from build123d import *
from OCP.BRepFilletAPI import BRepFilletAPI_MakeChamfer

# Parameters (mm, degrees)
SKETCH1_R             = 1.7
BOSS_EXTRUDE1_DEPTH   = 2
SKETCH2_W             = 30
SKETCH2_H             = 2
BOSS_EXTRUDE2_DEPTH   = 35
CUT_EXTRUDE1_DEPTH    = 2
SKETCH5_W             = 17
SKETCH5_H             = 15.5
CUT_EXTRUDE2_DEPTH    = 2
SKETCH6_R             = 1.2
CUT_EXTRUDE3_DEPTH    = 2
BOSS_EXTRUDE4_START   = -2
SKETCH7_W             = 30
SKETCH7_H             = 2
BOSS_EXTRUDE4_DEPTH   = 2
SKETCH8_W             = 20
SKETCH8_H             = 3
CUT_EXTRUDE4_DEPTH    = 2
SKETCH9_W             = 17
SKETCH9_H             = 3
CUT_EXTRUDE5_DEPTH    = 2
SKETCH10_W            = 2
SKETCH10_H            = 20
BOSS_EXTRUDE5_DEPTH   = 5
CUT_EXTRUDE6_START    = -30
CUT_EXTRUDE6_DEPTH    = 30
FILLET1_R             = 10
SKETCH12_W            = 20
SKETCH12_H            = 18.563508327
CUT_EXTRUDE7_DEPTH    = 2
FILLET2_R             = 2
BOSS_EXTRUDE6_START   = -2
BOSS_EXTRUDE6_DEPTH   = 2
BOSS_EXTRUDE7_START   = -2
SKETCH14_W            = 21
SKETCH14_H            = 11.5
BOSS_EXTRUDE7_DEPTH   = 2
BOSS_EXTRUDE8_START   = -2
BOSS_EXTRUDE8_DEPTH   = 2
FILLET3_R             = 2
FILLET4_R             = 6
SKETCH16_W            = 20
SKETCH16_H            = 8.5
CUT_EXTRUDE8_DEPTH    = 2
FILLET5_R             = 5
CHAMFER1_SIZE         = 2
CHAMFER1_SIZE2        = 2.748737084
CHAMFER1_SIZE2_2      = 2.596624047
CHAMFER2_SIZE         = 1
CHAMFER2_EDGE_2_SIZE  = 1
CHAMFER2_EDGE_3_SIZE  = 1
CHAMFER2_EDGE_3_SIZE2 = 2.732050808
CHAMFER2_EDGE_4_SIZE  = 1
CHAMFER2_EDGE_4_SIZE2 = 2.732050808
FILLET6_R             = 6


# Some blends are built 0.0001 mm under size
with BuildPart() as part:
    # Sketch1 → Boss-Extrude1 (new body)
    with BuildSketch(Plane(origin=(0, 0, 0), x_dir=(1, 0, 0), z_dir=(0, 1, 0))):
        with BuildLine():
            Line((-21.310608918, 0), (21.310608918, 0))
            ThreePointArc((21.310608918, 0), (26.45, 5.139391082), (31.589391082, 0))
            Line((31.589391082, 0), (31.589391082, -16))
            Line((31.589391082, -16), (10, -16))
            Line((10, -16), (10, -10.526162893))
            Line((10, -10.526162893), (10, -3))
            Line((10, -3), (-10, -3))
            Line((-10, -3), (-10, -10.526162893))
            Line((-10, -10.526162893), (-10, -16))
            Line((-10, -16), (-31.589391082, -16))
            Line((-31.589391082, -16), (-31.589391082, 0))
            ThreePointArc((-31.589391082, 0), (-26.45, 5.139391082), (-21.310608918, 0))
        make_face()
        with Locations(Location((-26.45, 0, 0), (0, 0, 270))):
            Circle(SKETCH1_R, mode=Mode.SUBTRACT)
        with Locations(Location((26.45, 0, 0), (0, 0, 270))):
            Circle(SKETCH1_R, mode=Mode.SUBTRACT)
    extrude(amount=BOSS_EXTRUDE1_DEPTH)

    # Sketch2 → Boss-Extrude2 (add)
    with BuildSketch(Plane(origin=(0, 2, 0), x_dir=(1, 0, 0), z_dir=(0, 1, 0))):
        with Locations((0, -15)):
            Rectangle(SKETCH2_W, SKETCH2_H)
    extrude(amount=BOSS_EXTRUDE2_DEPTH)

    # Sketch4 → Cut-Extrude1 (cut)
    with BuildSketch(Plane.XY.offset(16)):
        with BuildLine():
            Line((-12.5, 33), (-12.5, 24.5))
            Line((-12.5, 24.5), (-10.5, 24.5))
            ThreePointArc((-10.5, 24.5), (-9.085786438, 23.914213562), (-8.5, 22.5))
            Line((-8.5, 22.5), (-8.5, 20.5))
            Line((-8.5, 20.5), (8.5, 20.5))
            Line((8.5, 20.5), (8.5, 22.5))
            ThreePointArc((8.5, 22.5), (9.085786438, 23.914213562), (10.5, 24.5))
            Line((10.5, 24.5), (12.5, 24.5))
            Line((12.5, 24.5), (12.5, 33))
            Line((12.5, 33), (10.5, 33))
            ThreePointArc((10.5, 33), (9.085786438, 33.585786438), (8.5, 35))
            Line((8.5, 35), (8.5, 37))
            Line((8.5, 37), (-8.5, 37))
            Line((-8.5, 37), (-8.5, 35))
            ThreePointArc((-8.5, 35), (-9.085786438, 33.585786438), (-10.5, 33))
            Line((-10.5, 33), (-12.5, 33))
        make_face()
    extrude(amount=-CUT_EXTRUDE1_DEPTH, mode=Mode.SUBTRACT)

    # Sketch5 → Cut-Extrude2 (cut)
    with BuildSketch(Plane.XY.offset(16)):
        with Locations((0, 12.75)):
            Rectangle(SKETCH5_W, SKETCH5_H)
    extrude(amount=-CUT_EXTRUDE2_DEPTH, mode=Mode.SUBTRACT)

    # Sketch6 → Cut-Extrude3 (cut)
    with BuildSketch(Plane.XY.offset(16)):
        with Locations((-10.5, 35)):
            Circle(SKETCH6_R)
        with Locations((10.5, 35)):
            Circle(SKETCH6_R)
        with Locations((-10.5, 22.5)):
            Circle(SKETCH6_R)
        with Locations((10.5, 22.5)):
            Circle(SKETCH6_R)
    extrude(amount=-CUT_EXTRUDE3_DEPTH, mode=Mode.SUBTRACT)

    # Sketch7 → Boss-Extrude4 (add)
    with BuildSketch(Plane.XY.offset(16).offset(BOSS_EXTRUDE4_START)):
        with Locations((0, 38)):
            Rectangle(SKETCH7_W, SKETCH7_H)
    extrude(amount=BOSS_EXTRUDE4_DEPTH)

    # Sketch8 → Cut-Extrude4 (cut)
    with BuildSketch(Plane(origin=(0, 2, 0), x_dir=(1, 0, 0), z_dir=(0, 1, 0))):
        with Locations((0, -1.5)):
            Rectangle(SKETCH8_W, SKETCH8_H)
    extrude(amount=-CUT_EXTRUDE4_DEPTH, mode=Mode.SUBTRACT)

    # Sketch9 → Cut-Extrude5 (cut)
    with BuildSketch(Plane.XY.offset(16)):
        with Locations((0, 3.5)):
            Rectangle(SKETCH9_W, SKETCH9_H)
    extrude(amount=-CUT_EXTRUDE5_DEPTH, mode=Mode.SUBTRACT)

    # Sketch10 → Boss-Extrude5 (add)
    with BuildSketch(Plane(origin=(0, 0, 14), x_dir=(-1, 0, 0), z_dir=(0, 0, -1))):
        with Locations((14, 12)):
            Rectangle(SKETCH10_W, SKETCH10_H)
        with Locations((-14, 12)):
            Rectangle(SKETCH10_W, SKETCH10_H)
    extrude(amount=BOSS_EXTRUDE5_DEPTH)

    # Sketch11 → Cut-Extrude6 (cut)
    with BuildSketch(Plane.ZY.offset(15).offset(CUT_EXTRUDE6_START)):
        Polygon((14, 22), (9, 2), (9, 22), align=None)
    extrude(amount=CUT_EXTRUDE6_DEPTH, mode=Mode.SUBTRACT)

    # Fillet1
    fillet1_edges = [part.edges().sort_by_distance(p)[0] for p in [
        (31.589391082, 1, 16),
        (-31.589391082, 1, 16),
    ]]
    fillet(fillet1_edges, radius=FILLET1_R)

    # Sketch12 → Cut-Extrude7 (cut)
    with BuildSketch(Plane.XY.offset(16)):
        with Locations((0, 11.281754164)):
            Rectangle(SKETCH12_W, SKETCH12_H)
    extrude(amount=-CUT_EXTRUDE7_DEPTH, mode=Mode.SUBTRACT)

    # Fillet2
    # the kernel refuses this fillet: 2 mm, written as the material it takes off along each edge
    with BuildSketch(Plane(origin=(8.5, 20.563508327, 9.158770817), x_dir=(0, 1, 0), z_dir=(0, 0, 1))) as fillet2_piece_1:
        with BuildLine():
            CenterArc((1.936491673, -2), FILLET2_R, 90, 75.522487814)
            Line((0, -1.5), (-0.038729833, -1.49))
            ThreePointArc((-0.038729833, -1.49), (-0.04, -0.75), (-0.04, 0))
            Line((-0.04, 0), (0, 0.04))
            Line((0, 0.04), (1.936491673, 0.04))
            Line((1.936491673, 0.04), (1.936491673, 0))
        make_face()
    extrude(amount=11.682458366, mode=Mode.SUBTRACT)
    with BuildSketch(Plane(origin=(-8.5, 20.563508327, 9.158770817), x_dir=(-1, 0, 0), z_dir=(0, 0, 1))) as fillet2_piece_2:
        with BuildLine():
            CenterArc((2, -1.936491673), FILLET2_R, 104.477512186, 75.522487814)
            Line((0, -1.936491673), (-0.04, -1.936491673))
            Line((-0.04, -1.936491673), (-0.04, 0))
            Line((-0.04, 0), (0, 0.04))
            ThreePointArc((0, 0.04), (0.75, 0.04), (1.49, 0.038729833))
            Line((1.49, 0.038729833), (1.5, 0))
        make_face()
    extrude(amount=11.682458366, mode=Mode.SUBTRACT)

    # Sketch13 → Boss-Extrude6 (add)
    with BuildSketch(Plane.XY.offset(16).offset(BOSS_EXTRUDE6_START)):
        Polygon((-15, 2), (-15, 33), (-21.589391082, 2), align=None)
        Polygon((21.589391082, 2), (15, 2), (15, 33), align=None)
    extrude(amount=BOSS_EXTRUDE6_DEPTH)

    # Sketch14 → Boss-Extrude7 (add)
    with BuildSketch(Plane.XY.offset(16).offset(BOSS_EXTRUDE7_START)):
        with Locations((0, 10.75)):
            Rectangle(SKETCH14_W, SKETCH14_H)
    extrude(amount=BOSS_EXTRUDE7_DEPTH)

    # Sketch15 → Boss-Extrude8 (add)
    with BuildSketch(Plane.XY.offset(16).offset(BOSS_EXTRUDE8_START)):
        with BuildLine():
            Line((-8.5, 22.5), (-8.5, 16.5))
            Line((-8.5, 16.5), (-10, 16.5))
            Line((-10, 16.5), (-10, 20.563508327))
            ThreePointArc((-10, 20.563508327), (-8.91886117, 21.275255129), (-8.5, 22.5))
        make_face()
        with BuildLine():
            Line((8.5, 22.5), (8.5, 16.5))
            Line((8.5, 16.5), (10, 16.5))
            Line((10, 16.5), (10, 20.563508327))
            ThreePointArc((10, 20.563508327), (8.91886117, 21.275255129), (8.5, 22.5))
        make_face()
    extrude(amount=BOSS_EXTRUDE8_DEPTH)

    # Fillet3
    fillet3_edges = [part.edges().sort_by_distance(p)[0] for p in [
        (-8.5, 16.5, 15),
        (8.5, 16.5, 15),
        (12.5, 24.5, 15),
        (-12.5, 24.5, 15),
        (12.5, 33, 15),
        (8.5, 37, 15),
        (-8.5, 37, 15),
        (-12.5, 33, 15),
    ]]
    fillet(fillet3_edges, radius=FILLET3_R - 0.0001)  # a hair under: the kernel refuses the full size

    # Fillet4
    fillet4_edges = [part.edges().sort_by_distance(p)[0] for p in [
        (15, 39, 15),
        (-15, 39, 15),
    ]]
    fillet(fillet4_edges, radius=FILLET4_R - 0.0001)  # a hair under: the kernel refuses the full size

    # Sketch16 → Cut-Extrude8 (cut)
    with BuildSketch(Plane.XY.offset(16)):
        with Locations((0, 9.25)):
            Rectangle(SKETCH16_W, SKETCH16_H)
    extrude(amount=-CUT_EXTRUDE8_DEPTH, mode=Mode.SUBTRACT)

    # Fillet5
    fillet5_edges = [part.edges().sort_by_distance(p)[0] for p in [
        (-10, 13.5, 15),
        (10, 13.5, 15),
    ]]
    fillet(fillet5_edges, radius=FILLET5_R)

    # Chamfer1: one chamfer whose edges measure the first distance from different faces: ONE call of the kernel's chamfer builder (chamfer() names one face for all edges)
    chamfer1_edges_1 = [part.edges().sort_by_distance(p)[0] for p in [
        (-13, 2, 11.5),
        (11.5, 2, 14),
        (13, 2, 11.5),
        (-18.294695541, 2, 14),
        (15, 2, 11.5),
        (18.294695541, 2, 14),
        (-11.5, 2, 14),
        (-15, 2, 11.5),
    ]]
    chamfer1_edges_2 = [part.edges().sort_by_distance(p)[0] for p in [
        (-14, 2, 9),
    ]]
    chamfer1_side_2 = [part.faces().sort_by_distance(p)[0] for p in [
        (-21.362181676, 2, 5.92457091),
    ]]
    chamfer1_edges_3 = [part.edges().sort_by_distance(p)[0] for p in [
        (14, 2, 9),
    ]]
    chamfer1_side_3 = [part.faces().sort_by_distance(p)[0] for p in [
        (21.362181676, 2, 5.92457091),
    ]]
    chamfer1_edges_4 = [part.edges().sort_by_distance(p)[0] for p in [
        (-21.589391082, 2, 15),
    ]]
    chamfer1_side_4 = [part.faces().sort_by_distance(p)[0] for p in [
        (-21.362181676, 2, 5.92457091),
    ]]
    chamfer1_edges_5 = [part.edges().sort_by_distance(p)[0] for p in [
        (21.589391082, 2, 15),
    ]]
    chamfer1_side_5 = [part.faces().sort_by_distance(p)[0] for p in [
        (18.294695541, 17.5, 15),
    ]]
    chamfer1 = BRepFilletAPI_MakeChamfer(part.part.solid().wrapped)
    for e in chamfer1_edges_1:
        chamfer1.Add(CHAMFER1_SIZE, e.wrapped)
    for e in chamfer1_edges_2:
        chamfer1.Add(CHAMFER1_SIZE, CHAMFER1_SIZE2, e.wrapped, chamfer1_side_2[0].wrapped)  # the first distance lies on this face
    for e in chamfer1_edges_3:
        chamfer1.Add(CHAMFER1_SIZE, CHAMFER1_SIZE2, e.wrapped, chamfer1_side_3[0].wrapped)  # the first distance lies on this face
    for e in chamfer1_edges_4:
        chamfer1.Add(CHAMFER1_SIZE, CHAMFER1_SIZE2_2, e.wrapped, chamfer1_side_4[0].wrapped)  # the first distance lies on this face
    for e in chamfer1_edges_5:
        chamfer1.Add(CHAMFER1_SIZE, CHAMFER1_SIZE2_2, e.wrapped, chamfer1_side_5[0].wrapped)  # the first distance lies on this face
    add(Compound.cast(chamfer1.Shape()), mode=Mode.REPLACE)

    # Chamfer2
    chamfer2_edges = [part.edges().sort_by_distance(p)[0] for p in [
        (15, 13, 14),
    ]]
    chamfer(chamfer2_edges, length=CHAMFER2_SIZE)

    # Chamfer2 edge 2
    chamfer2_edge_2_edges = [part.edges().sort_by_distance(p)[0] for p in [
        (-15, 13, 14),
    ]]
    chamfer(chamfer2_edge_2_edges, length=CHAMFER2_EDGE_2_SIZE)

    # Chamfer2 edge 3
    chamfer2_edge_3_edges = [part.edges().sort_by_distance(p)[0] for p in [
        (16, 3, 13),
    ]]
    chamfer2_edge_3_side = [part.faces().sort_by_distance(p)[0] for p in [
        (19.357625286, 2.973019207, 12.973019207),
    ]]
    chamfer(chamfer2_edge_3_edges, length=CHAMFER2_EDGE_3_SIZE, length2=CHAMFER2_EDGE_3_SIZE2, reference=chamfer2_edge_3_side[0])

    # Chamfer2 edge 4
    chamfer2_edge_4_edges = [part.edges().sort_by_distance(p)[0] for p in [
        (-16, 3, 13),
    ]]
    chamfer2_edge_4_side = [part.faces().sort_by_distance(p)[0] for p in [
        (-19.294695541, 3, 13),
    ]]
    chamfer(chamfer2_edge_4_edges, length=CHAMFER2_EDGE_4_SIZE, length2=CHAMFER2_EDGE_4_SIZE2, reference=chamfer2_edge_4_side[0])

    # Fillet6
    fillet6_edges = [part.edges().sort_by_distance(p)[0] for p in [
        (-10, 1, 0),
        (10, 1, 0),
    ]]
    fillet(fillet6_edges, radius=FILLET6_R)


solid = part.part
CAD build for the part. Positions are in the model's coordinates, mm. A direction names the side the tool comes from. Coordinates: 2 decimals unless noted, no trailing zeros. Write each loop counter-clockwise with the first axis right and the second up, starting at its lowest first coordinate (ties: lowest second). Pieces come first, ordered by that corner, then holes. Notation, with made-up numbers: (55, 2) - (90, 2) arc R34 cw to (90, 34) - close; hole circle Ø2 at (82, 2.5). An arc over 180 degrees is marked (long way). Use a Markdown table: item, result. Add a question column.
Item 1: Drill centre lines: L1, parallel to Y at x = -10.5, z = 15.5; L2, parallel to Z at x = -18, y = 13.5; L3, parallel to Y at x = -11, z = 7. Where is each one in solid material? Low to high. Write a range as from..to.
Item 2: Flat gauge pins, fed straight in: pin 1 (10 mm diameter, centred on x = -3, y = 6.5, fed in from -Z); pin 2 (3 mm diameter, centred on x = -10.5, y = 35, fed in from +Z); pin 3 (1.6 mm diameter, centred on y = 29.5, z = 14.5, fed in from +X); pin 4 (2 mm diameter, centred on x = 19, y = 1, fed in from -Z). Where does each tip first touch, or does it go through?
Item 3: Band-saw the part on B-B, the plane y = 6. Give the cut face in (x, z).
Item 4: 3-axis set-ups, long thin cutter, end or side, ignore diameter. For faces 5 (the face through (-13, 9, 13)), 6 (the face through (0, 13.5, 15)), 7 (the face through (-7.93, 17.1, 15.01)), 8 (the face through (13.196, 37.289, 15.014)): which of +Z, -Z, +X, -X, +Y, -Y reach the whole face in a straight line?
Item 5: Mould opens along X. For faces 1 (the face through (-11.9, 25.07, 14.99)), 2 (the face through (-13.289, 37.196, 15.014)), 3 (the face through (-11.711, 0.986, 1.804)), 4 (the face through (22.701, 2.964, 14.416)) say: pulls with the +X half, pulls with the -X half, needs draft (parallel to the pull), parting line crosses it, or undercut.
Item 6: Band-saw the part on D-D, the plane x = -26.45. Give the cut face in (y, z), and give its area (3 significant figures).
Item 7: Band-saw the part on A-A, the plane x = -1. Give the cut face in (y, z), and give its area (3 significant figures).
Item 8: Band-saw the part on C-C, the plane y = 10.5. Give the cut face in (x, z) (3 decimals).
Numbers:
| question | item | result |
|---|---|---|
| 1 | L1 | 0..21.3, 23.7..24.5, 33..33.8, 36.2..38.81 |
| 1 | L2 | 14..16 |
| 1 | L3 | 0..2 |
| 2 | pin 1 | through |
| 2 | pin 2 | z = 16 |
| 2 | pin 3 | x = 15.91 |
| 2 | pin 4 | z = 0 |
| 3 | outline | (-20.74, 14) - (-16, 14) - (-15, 13) - (-15, 10) - (-13, 10) - (-13, 14) - (-10, 14) - (-10, 16) - (-20.74, 16) - close; (10, 14) - (13, 14) - (13, 10) - (15, 10) - (15, 13) - (16, 14) - (20.74, 14) - (20.74, 16) - (10, 16) - close |
| 4 | face 5 | -Z, +Y |
| 4 | face 6 | +Z, -Z, -Y |
| 4 | face 7 | +Z, -Z |
| 4 | face 8 | +Z, -Z, +X, +Y |
| 5 | face 1 | undercut |
| 5 | face 2 | pulls with the -X half |
| 5 | face 3 | undercut |
| 5 | face 4 | pulls with the +X half |
| 6 | outline | (0, -5.14) - (2, -5.14) - (2, -1.7) - (0, -1.7) - close; (0, 1.7) - (2, 1.7) - (2, 14.74) - (0, 14.74) - close |
| 6 | area | 33.0 mm2 |
| 7 | outline | (13.5, 14) - (16.5, 14) - (16.5, 16) - (13.5, 16) - close; (37, 14) - (39, 14) - (39, 16) - (37, 16) - close |
| 7 | area | 10.0 mm2 |
| 8 | outline | (-19.783, 14) - (-16, 14) - (-15, 13) - (-15, 11.125) - (-13, 11.125) - (-13, 14) - (-9.583, 14) - (-9.583, 16) - (-19.783, 16) - close; (9.583, 14) - (13, 14) - (13, 11.125) - (15, 11.125) - (15, 13) - (16, 14) - (19.783, 14) - (19.783, 16) - (9.583, 16) - close |
